Source: CAD feature listing. Evaluate the final solid. Frame: model axes, mm. Face numbers are marked on the shaded views. A direction names the side the tool comes from. Coordinates: 2 decimals unless noted, no trailing zeros. Loops run counter-clockwise (first coordinate to the right, second up) from the corner with the lowest first, then second, coordinate; pieces in that order, holes last. Notation, with made-up numbers: M 63.25,59.25 L 95.25,59.25 A13 cw 95.25,64.25 Z; hole C 24.5,-8.5 d2. An arc over 180 degrees is marked long. One line per question, with ' | ' between items. Start each with the question number.
1. Section query C-C, the plane y = -4.5. Output: boundary loops of the cut face in (x, z).
2. Section query B-B, the plane x = 0. Output: boundary loops of the cut face in (y, z), and give its area (3 significant figures).
3. Section query A-A, the plane z = 0. Output: boundary loops of the cut face in (x, y), and give its area (3 significant figures).
4. Mould query, pull axis Z, two halves, no side actions, for the marked faces 1 and 2. Classes: pulls with the +Z half, pulls with the -Z half, needs draft (parallel to the pull), parting line crosses it, or undercut.
5. Section query D-D, the plane z = -19. Output: boundary loops of the cut face in (x, y) (3 decimals), and give its area (3 significant figures).
6. Ray query, probe 1 along Z at (x, y) = (0, -0.3); probe 2 along Z at (x, y) = (0, 0.2); probe 3 along Y at (x, z) = (-29, 3.5). Return the intervals inside material, ascending.
7. Pin query (flat end, axial travel): P1, Ø21, axis at x = 9, z = -2.5, coming from the -Y side; P2, Ø1.5, axis at y = -3.5, z = 17.5, coming from the +X side; P3, Ø1.5, axis at y = -0.5, z = 1, coming from the +X side; P4, Ø2, axis at y = -2, z = -2, coming from the +X side. Return the tip coordinate at first contact, or that it passes through.
8. Access query for the marked faces 3 and 4. Directions: +Z, -Z, +X, -X, +Y, -Y. A direction counts if a zero-diameter tool reaches every point of the face in a straight line with its end or side. Return the directions, or none.
Autodesk Inventor part; units mm, degrees
ref_plane "YZ Plane" through (0, 0, 0) normal (1, 0, 0) x (0, 1, 0)
ref_plane "XZ Plane" through (0, 0, 0) normal (0, 1, 0) x (-1, 0, 0)
ref_plane "XY Plane" through (0, 0, 0) normal (0, 0, 1) x (1, 0, 0)
sketch "Sketch1" plane through (0, 0, 0) normal (0, 1, 0) x (-1, 0, 0)
  circle A0 centre (0, 0) radius 32
  dimension "d0" = 64
extrude "Extrusion1" add sketch "Sketch1" along normal blind 2
sketch "Sketch2" plane through (0, 0, 0) normal (0, -1, 0) x (1, 0, 0)
  circle A0 centre (0, 0) radius 20.75
  circle A1 centre (0, 0) radius 20
  dimension "d3" = 41.5
  dimension "d4" = 40
extrude "Extrusion2" add sketch "Sketch2" along normal blind 2
sketch "Sketch3" plane through (0, 0, 0) normal (0, -1, 0) x (1, 0, 0)
  circle A0 centre (0, 0) radius 20
extrude "Extrusion3" cut sketch "Sketch3" against normal blind 2
sketch "Sketch4" plane through (0, 0, 0) normal (0, -1, 0) x (1, 0, 0)
  circle A0 centre (19, 19) radius 2.75
  point P0 (0, 0)
  dimension "d9" = 5.5
  dimension "d10" = 19
  dimension "d11" = 19
extrude "Extrusion4" add sketch "Sketch4" along normal blind 6.5
pattern_circular "Circular Pattern1" count 4 over 360 about axis through (0, -10, 0) along (0, 1, 0) of "Extrusion4"
properties part number "pot_base_adapter1"
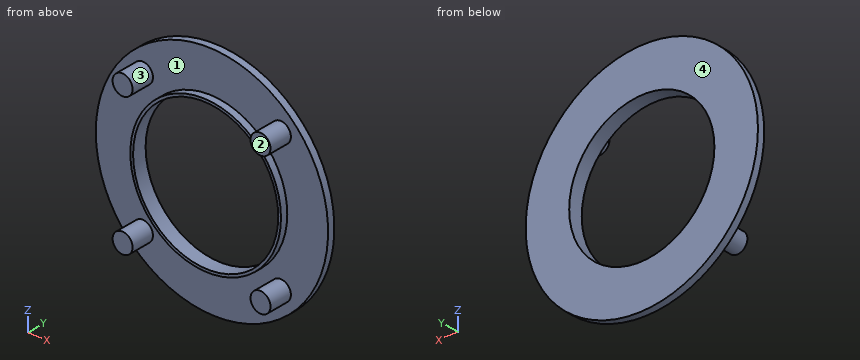
Taken from the geometry:
1) outline: C -19,-19 d5.5; C -19,19 d5.5; C 19,-19 d5.5; C 19,19 d5.5
2) outline: M -2,-20.75 L 0,-20.75 L 0,-32 L 2,-32 L 2,-20 L -2,-20 Z; M -2,20 L 2,20 L 2,32 L 0,32 L 0,20.75 L -2,20.75 Z | area: 51.0 mm^2
3) outline: M -32,0 L -20.75,0 L -20.75,-2 L -20,-2 L -20,2 L -32,2 Z; M 20,-2 L 20.75,-2 L 20.75,0 L 32,0 L 32,2 L 20,2 Z | area: 51.0 mm^2
4) face 1: undercut | face 2: needs draft
5) outline: M -25.749,0 L -21.75,0 L -21.75,-6.5 L -16.25,-6.5 L -16.25,0 L -8.34,0 L -8.34,-2 L -6.245,-2 L -6.245,2 L -25.749,2 Z; M 6.245,-2 L 8.34,-2 L 8.34,0 L 16.25,0 L 16.25,-6.5 L 21.75,-6.5 L 21.75,0 L 25.749,0 L 25.749,2 L 6.245,2 Z | area: 158 mm^2
6) probe 1: -20.75 to -20, 20 to 20.75 | probe 2: -32 to -20, 20 to 32 | probe 3: 0 to 2
7) P1: through | P2: x = 21.65 | P3: x = 32 | P4: x = 20.73
8) face 3: -Y | face 4: +Z, -Z, +X, -X, +Y
